Check sheet for the modelled part. Datum: model origin and axes. Units: mm. Face numbers are marked on the shaded views. A direction names the side the tool comes from. Coordinates: 2 decimals unless noted, no trailing zeros. Loops run counter-clockwise (first coordinate to the right, second up) from the corner with the lowest first, then second, coordinate; pieces in that order, holes last.
```python
from build123d import *

# Parameters (mm, degrees)
ESQUISSE1_W             = 12
ESQUISSE1_H             = 12
BOSS_EXTRU_1_DEPTH      = 3
BOSS_EXTRU_2_DEPTH      = 0.2
BOSS_EXTRU_3_DEPTH      = 1
ESQUISSE4_W             = 0.2
ESQUISSE4_H             = 2
BOSS_EXTRU_4_DEPTH      = 0.1
ESQUISSE5_R             = 4
BOSS_EXTRU_5_DEPTH      = 2
ESQUISSE6_R             = 3.5
ENL_V_MAT_EXTRU_1_DEPTH = 2
ESQUISSE7_R             = 3.5
BOSS_EXTRU_6_DEPTH      = 3


with BuildPart() as part:
    # Esquisse1 → Boss.-Extru.1 (new body)
    with BuildSketch(Plane.XY):
        Rectangle(ESQUISSE1_W, ESQUISSE1_H)
    extrude(amount=BOSS_EXTRU_1_DEPTH)

    # Esquisse2 → Boss.-Extru.2 (add)
    with BuildSketch(Plane.XY.offset(3)):
        Polygon((-5.5, 1), (-5.5, 5.5), (5.5, 5.5), (5.5, 1), (7.5, 1), (7.5, -1), (5.5, -1), (5.5, -5.5), (-5.5, -5.5), (-5.5, -1), (-7.5, -1), (-7.5, 1), align=None)
    extrude(amount=BOSS_EXTRU_2_DEPTH)

    # Esquisse3 → Boss.-Extru.3 (add, symmetric)
    with BuildSketch(Plane(origin=(0, 0, 0), x_dir=(1, 0, 0), z_dir=(0, 1, 0))):
        Polygon((6, -3), (6, -2.5), (6.75, -2.5), (6.75, -2), (7.5, -2), (7.5, -3), align=None)
        Polygon((-7.5, -3), (-6, -3), (-6, -2.5), (-6.75, -2.5), (-6.75, -2), (-7.5, -2), align=None)
    extrude(amount=BOSS_EXTRU_3_DEPTH, both=True)

    # Esquisse4 → Boss.-Extru.4 (add, symmetric)
    with BuildSketch(Plane(origin=(0, 0, 0), x_dir=(1, 0, 0), z_dir=(0, 1, 0))):
        with Locations((7.125, -1)):
            Rectangle(ESQUISSE4_W, ESQUISSE4_H)
        with Locations((-7.125, -1)):
            Rectangle(ESQUISSE4_W, ESQUISSE4_H)
    extrude(amount=BOSS_EXTRU_4_DEPTH, both=True)

    # Esquisse5 → Boss.-Extru.5 (add)
    with BuildSketch(Plane.XY.offset(3.2)):
        Circle(ESQUISSE5_R)
    extrude(amount=BOSS_EXTRU_5_DEPTH)

    # Esquisse6 → Enlèv. mat.-Extru.1 (cut)
    with BuildSketch(Plane.XY.offset(5.2)):
        Circle(ESQUISSE6_R)
    extrude(amount=-ENL_V_MAT_EXTRU_1_DEPTH, mode=Mode.SUBTRACT)

    # Esquisse7 → Boss.-Extru.6 (add)
    with BuildSketch(Plane.XY.offset(3.2)):
        Circle(ESQUISSE7_R)
    extrude(amount=BOSS_EXTRU_6_DEPTH)


solid = part.part
```
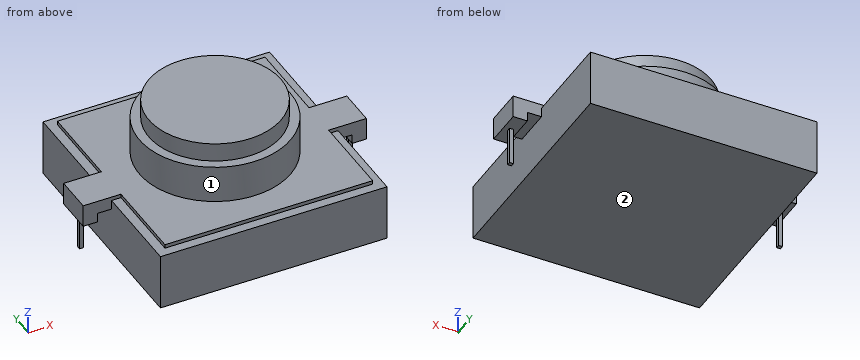
1) Section check B-B on x = 4.5. Enter the section's corners in (y, z).
Answer sheet:
outline: (-6, 0) - (6, 0) - (6, 3) - (5.5, 3) - (5.5, 3.2) - (-5.5, 3.2) - (-5.5, 3) - (-6, 3) - close
2) Section check C-C on y = -2. Enter the section's corners in (x, z), plus the area to 3 significant figures.
Answer sheet:
outline: (-6, 0) - (6, 0) - (6, 3) - (5.5, 3) - (5.5, 3.2) - (3.46, 3.2) - (3.46, 5.2) - (2.87, 5.2) - (2.87, 6.2) - (-2.87, 6.2) - (-2.87, 5.2) - (-3.46, 5.2) - (-3.46, 3.2) - (-5.5, 3.2) - (-5.5, 3) - (-6, 3) - close
area: 57.8 mm2
3) Section check D-D on x = 0. Enter the section's corners in (y, z), plus the area to 3 significant figures.
Answer sheet:
outline: (-6, 0) - (6, 0) - (6, 3) - (5.5, 3) - (5.5, 3.2) - (4, 3.2) - (4, 5.2) - (3.5, 5.2) - (3.5, 6.2) - (-3.5, 6.2) - (-3.5, 5.2) - (-4, 5.2) - (-4, 3.2) - (-5.5, 3.2) - (-5.5, 3) - (-6, 3) - close
area: 61.2 mm2
4) Scan lines: line 1 (Z direction, x = -4, y = 0.75); line 2 (X direction, y = 3, z = 0.5); line 3 (Z direction, x = -3.5, y = 0.75). Record each from-to range of solid material in increasing order.
Answer sheet:
line 1: z = 0 to 3.2
line 2: x = -6 to 6
line 3: z = 0 to 5.2
5) Section check A-A on z = 1.5. Enter the section's corners in (x, y) (3 decimals), plus the area to 3 significant figures.
Answer sheet:
outline: (-7.225, -0.1) - (-7.025, -0.1) - (-7.025, 0.1) - (-7.225, 0.1) - close; (-6, -6) - (6, -6) - (6, 6) - (-6, 6) - close; (7.025, -0.1) - (7.225, -0.1) - (7.225, 0.1) - (7.025, 0.1) - close
area: 144 mm2
6) Depth check by flat-ended pin: pin 1 (1.5 mm diameter, centred on x = -0.5, y = 4.5, fed in from -Z); pin 2 (2 mm diameter, centred on x = 1.5, z = 5, fed in from -Y); pin 3 (0.6 mm diameter, centred on x = 6.5, y = -0.5, fed in from -Z); pin 4 (0.6 mm diameter, centred on x = -7, z = 2.5, fed in from -Y). Enter the tip coordinate at first touch or a pass-through.
Answer sheet:
pin 1: stops at z = 0
pin 2: stops at y = -3.97
pin 3: stops at z = 2
pin 4: stops at y = -1
7) Set-up check for the marked faces 1 and 2: record each of +Z, -Z, +X, -X, +Y, -Y from which the full face is reachable in a straight line by a thin tool's end or side.
Answer sheet:
face 1: +Z
face 2: -Z, +X, -X, +Y, -Y
